Could you check a few things on this model? Use its own coordinates, in mm. A direction names the side the tool comes from. Round coordinates to 2 decimals unless told otherwise and drop trailing zeros. Write each loop counter-clockwise with the first axis right and the second up, starting at its lowest first coordinate (ties: lowest second). Pieces come first, ordered by that corner, then holes. Notation, with made-up numbers: (-19.75, -4) -> (-1.75, -4) arc R25 ccw to (-1.75, 32) -> close; hole circle Ø3 at (-35, 25.5). An arc over 180 degrees is marked (long way). Answer in a Markdown table with one row per item. Add a question column.
```python
from build123d import *

# Parameters (mm, degrees)
F0_W     = 50.8
F0_H     = 19.05
F1_DEPTH = 774.7
F2_W     = 122.43557321
F2_H     = 50.8
F2_W_2   = 343.1604206562
F2_W_3   = 296.3738366961
F3_DEPTH = 25.4
F4_R     = 0.79375
F5_DEPTH = 25.4
F6_R     = 4.7625
F7_DEPTH = 25.4


# Not quite as in the source:
# - a feature names something its author has since deleted; it is built from what else it names


with BuildPart() as f1:
    # F0 (on Top) → F1 (new body)
    with BuildSketch(Plane.XY):
        Rectangle(F0_W, F0_H)
    extrude(amount=F1_DEPTH)

    # F2 (on Front) → F3 (cut)
    with BuildSketch(Plane.XZ):
        with Locations((22.4465244144, 25.4)):
            Rectangle(F2_W, F2_H)
        with Locations((-38.7818217278, 749.3)):
            Rectangle(F2_W_2, F2_H)
        with Locations((-46.0684634745, 361.95)):
            Rectangle(F2_W_3, F2_H)
    extrude(amount=F3_DEPTH, mode=Mode.SUBTRACT)

    # F4 (on Front) → F5 (cut)
    with BuildSketch(Plane.XZ):
        with Locations((9.525, 101.6)):
            Circle(F4_R)
        with Locations((9.525, 155.575)):
            Circle(F4_R)
        with Locations((9.525, 517.525)):
            Circle(F4_R)
        with Locations((9.525, 571.5)):
            Circle(F4_R)
        with Locations((-9.525, 517.525)):
            Circle(F4_R)
        with Locations((-9.525, 571.5)):
            Circle(F4_R)
        with Locations((-9.525, 101.6)):
            Circle(F4_R)
        with Locations((-9.525, 155.575)):
            Circle(F4_R)
    extrude(amount=-F5_DEPTH, mode=Mode.SUBTRACT)

    # F6 (on Front) → F7 (cut)
    with BuildSketch(Plane.XZ):
        with Locations((0, 95.25)):
            Circle(F6_R)
        with Locations((0, 361.95)):
            Circle(F6_R)
    extrude(amount=F7_DEPTH, mode=Mode.SUBTRACT)


solid = f1.part
```
(1) For P1, Ø7.5, axis at x = -11, y = -6.5, coming from the -Z side; P2, Ø0.5, axis at x = 9.5, z = 571.5, coming from the +Y side; P3, Ø10, axis at x = -10, y = 2.5, coming from the -Z side; P4, Ø3, axis at x = 0.5, z = 97.5, coming from the -Y side, each with a flat end and sliding along its axis, tell me the tip position at first contact or that it passes through.
(2) Suppose I cut it at A-A, the plane z = 348. Please give me the cut outline in (x, y) (3 decimals), then the cut area to 3 significant figures.
(3) I need wall thicknesses on L1, parallel to X at y = 3.25, z = 571.5; L2, parallel to Z at x = -5, y = -1; L3, parallel to X at y = -7, z = 95.25. Which ranges of each line are inside material? Lowest first, please.
(4) On a 3-axis mill with a long thin cutter (end or side, diameter ignored), from which of +Z, -Z, +X, -X, +Y, -Y can I reach the whole of each face in a straight line? I mean faces 1 (the face through (0, 0, 26)), 2 (the face through (0, 9.525, 382)), 3 (the face through (0, 0, 362)), 4 (the face through (0, 0, 750)). Say none if no direction works.
Response:
| question | item | result |
|---|---|---|
| 1 | P1 | z = 50.8 |
| 1 | P2 | y = 0 |
| 1 | P3 | z = 0 |
| 1 | P4 | y = 0 |
| 2 | outline | (-25.4, 0) -> (25.4, 0) -> (25.4, 9.525) -> (-25.4, 9.525) -> close |
| 2 | area | 484 mm² |
| 3 | L1 | -25.4 to -10.32, -8.73 to 8.73, 10.32 to 25.4 |
| 3 | L2 | 50.8 to 336.55, 387.35 to 723.9 |
| 3 | L3 | -25.4 to -4.76, 4.76 to 25.4 |
| 4 | face 1 | -Z, +X, -X, -Y |
| 4 | face 2 | +Z, -Z, +X, -X, +Y |
| 4 | face 3 | +X, -X, -Y |
| 4 | face 4 | +Z, +X, -X, -Y |
